from build123d import *

# Parameters (mm, degrees)
SKETCH1_R           = 1.55
BOSS_EXTRUDE1_DEPTH = 2
CHAMFER1_SIZE       = 0.1


with BuildPart() as part:
    # Sketch1 → Boss-Extrude1 (new body)
    with BuildSketch(Plane.XY):
        with BuildLine():
            Line((-12.5, 2.5), (12.5, 2.5))
            ThreePointArc((12.5, 2.5), (15, 0), (12.5, -2.5))
            Line((12.5, -2.5), (-12.5, -2.5))
            ThreePointArc((-12.5, -2.5), (-15, 0), (-12.5, 2.5))
        make_face()
        with Locations((-12.5, 0)):
            Circle(SKETCH1_R, mode=Mode.SUBTRACT)
        with Locations((12.5, 0)):
            Circle(SKETCH1_R, mode=Mode.SUBTRACT)
    extrude(amount=BOSS_EXTRUDE1_DEPTH)

    # Chamfer1
    chamfer1_edges = [part.edges().sort_by_distance(p)[0] for p in [
        (-14.05, 0, 0),
        (-14.05, 0, 2),
        (15, 0, 2),
        (10.95, 0, 0),
        (10.95, 0, 2),
        (0, 2.5, 2),
        (-15, 0, 2),
        (0, 2.5, 0),
        (15, 0, 0),
        (0, -2.5, 0),
        (-15, 0, 0),
        (0, -2.5, 2),
    ]]
    chamfer(chamfer1_edges, length=CHAMFER1_SIZE)


solid = part.part
For this review, take the finished solid that the model builds, in its own axes (mm). Give positions to 0.01 mm unless a question says otherwise; leave off trailing zeros. Order: outer loops, then holes, each group sorted by start corner. A loop starts at its lowest first (then second) coordinate and runs counter-clockwise, first axis right, second up. Notation, with made-up numbers: (-5.75, -14.5) -> (2.25, -14.5) arc R30 ccw to (2.25, 15.5) -> close; hole circle Ø3 at (20.5, 1). An arc over 180 degrees is marked (long way). Write item = value, one per line.
1) We need section A-A, the plane y = 0. Give the boundary of the cut face in (x, z).
Findings:
outline = (-15, 0.1) -> (-14.9, 0) -> (-14.15, 0) -> (-14.05, 0.1) -> (-14.05, 1.9) -> (-14.15, 2) -> (-14.9, 2) -> (-15, 1.9) -> close; (-10.95, 0.1) -> (-10.85, 0) -> (10.85, 0) -> (10.95, 0.1) -> (10.95, 1.9) -> (10.85, 2) -> (-10.85, 2) -> (-10.95, 1.9) -> close; (14.05, 0.1) -> (14.15, 0) -> (14.9, 0) -> (15, 0.1) -> (15, 1.9) -> (14.9, 2) -> (14.15, 2) -> (14.05, 1.9) -> close
2) Draft analysis for pull direction X (two halves, no side actions). For faces 1 (the face through (0, 0, 2)), 2 (the face through (11.27, -0.94, 0.99)), 3 (the face through (-15, 0, 1)), state which applies: pulls with the +X half, pulls with the -X half, needs draft (parallel to the pull), parting line crosses it, or undercut.
Findings:
face_1 = needs draft
face_2 = undercut
face_3 = pulls with the -X half
3) We need section B-B, the plane z = 1.3. Give the boundary of the cut face in (x, y).
Findings:
outline = (-12.5, -2.5) -> (12.5, -2.5) arc R2.5 ccw to (12.5, 2.5) -> (-12.5, 2.5) arc R2.5 ccw to start; hole circle Ø3.1 at (-12.5, 0); hole circle Ø3.1 at (12.5, 0)
4) Insertion check: pin 1 (1 mm diameter, centred on y = 1, z = 1, fed in from +X); pin 2 (2.5 mm diameter, centred on x = 12.5, y = 0, fed in from +Z). Each pin has a flat end and moves straight along its axis. Give the tip position at first contact, or say it passes through.
Findings:
pin_1 = 14.95
pin_2 = through
5) To check wall thickness, follow L1, parallel to Y at x = 12.5, z = 1.25; L2, parallel to X at y = -1.35, z = 0.5; L3, parallel to X at y = -0.35, z = 0.4. State the ranges of each line that lie inside material, in increasing order. Write a range as from..to.
Findings:
L1 = -2.5..-1.55, 1.55..2.5
L2 = -14.6..-13.26, -11.74..11.74, 13.26..14.6
L3 = -14.98..-14.01, -10.99..10.99, 14.01..14.98
